Design review of the part shown in the three views and the two pictorial views. Dimensions are in mm from the part's minimum x, y and z. A direction names the side the tool comes from. Round coordinates to 2 decimals unless told otherwise and drop trailing zeros. Loops run counter-clockwise (first coordinate to the right, second up) from the corner with the lowest first, then second, coordinate; pieces in that order, holes last. Notation, with made-up numbers: M 41.5,72 L 61.5,72 A37 cw 61.5,109 Z; hole C -39,70.5 d8. An arc over 180 degrees is marked long. One line per question, with ' | ' between items.
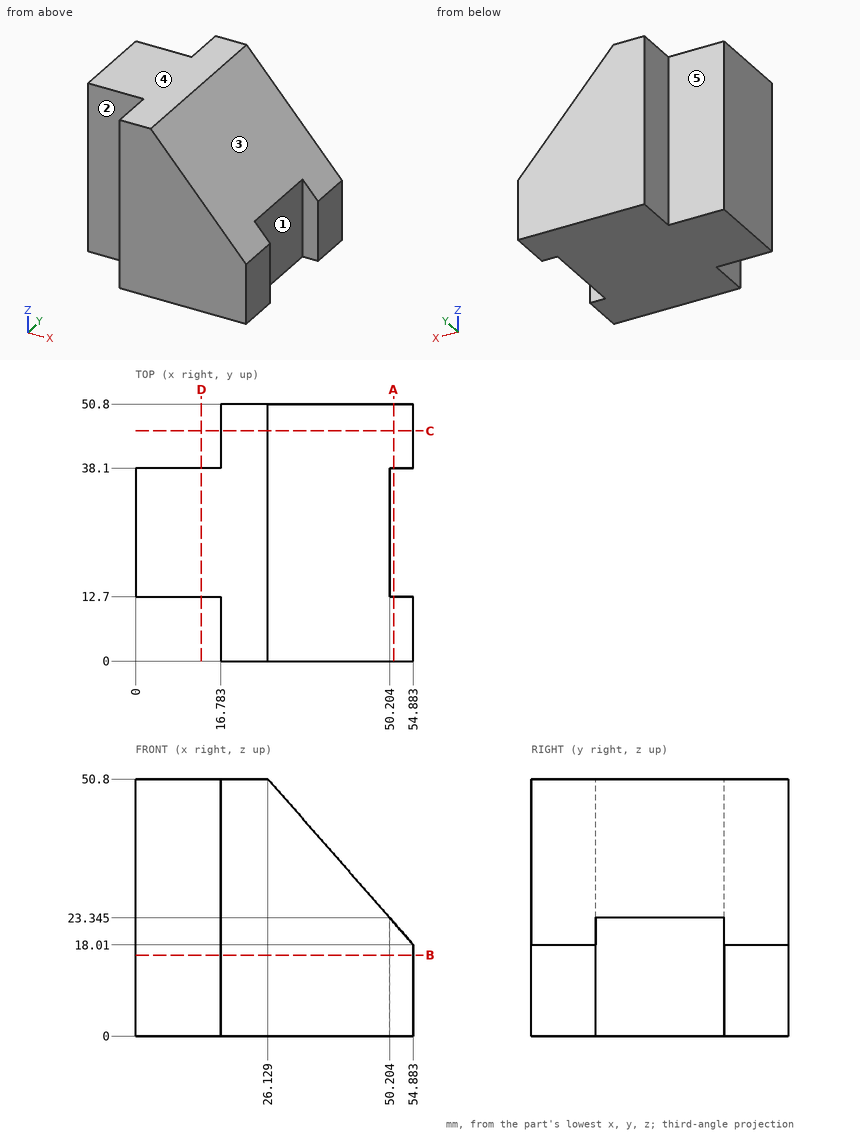
1) Add section C-C on y = 45.5. State the section outline as (x, z) points.
Output values:
outline: M 16.78,0 L 54.88,0 L 54.88,18.01 L 26.13,50.8 L 16.78,50.8 Z
2) Add section B-B on z = 16. State the section outline as (x, y) points, then the cut area to 3 significant figures.
Output values:
outline: M 0,12.7 L 16.78,12.7 L 16.78,0 L 54.88,0 L 54.88,12.7 L 50.2,12.7 L 50.2,38.1 L 54.88,38.1 L 54.88,50.8 L 16.78,50.8 L 16.78,38.1 L 0,38.1 Z | area: 2,240 mm²
3) Machinability: for the marked faces 4 and 5, which of the approach directions +Z, -Z, +X, -X, +Y, -Y give a long, thin tool a straight path to every point of the face, cutting with its end or side? Answer none if there is none.
Output values:
face 4: +Z, +X, -X, +Y, -Y | face 5: +Z, -Z, -X, +Y
4) Add section D-D on x = 13. State the section outline as (y, z) points, then the cut area to 3 significant figures.
Output values:
outline: M 12.7,0 L 38.1,0 L 38.1,50.8 L 12.7,50.8 Z | area: 1,290 mm²
5) Add section A-A on x = 51. State the section outline as (y, z) points, then the cut area to 3 significant figures.
Output values:
outline: M 0,0 L 12.7,0 L 12.7,22.44 L 0,22.44 Z; M 38.1,0 L 50.8,0 L 50.8,22.44 L 38.1,22.44 Z | area: 570 mm²
6) Insertion check: P1, Ø18.5, axis at y = 26, z = 15.5, coming from the +X side; P2, Ø10, axis at x = 9.5, z = 34.5, coming from the -Y side; P3, Ø1, axis at x = 42.5, y = 39.5, coming from the +Z side. Each pin has a flat end and moves straight along its axis. Give the tip position at first contact, or say it passes through.
Output values:
P1: stops at x = 50.2 | P2: stops at y = 12.7 | P3: stops at z = 32.7
7) For line 1 (X direction, y = 40.5, z = 12); line 2 (Y direction, x = 7, z = 6); line 3 (X direction, y = 16.5, z = 14.5), list the stretches that pass through material, from the lowest coordinate up.
Output values:
line 1: x = 16.78 to 54.88 | line 2: y = 12.7 to 38.1 | line 3: x = 0 to 50.2
8) Mouldability with a two-part tool opening along Y and no side actions: class the marked faces 1, 2 and 3 as +Y half, -Y half, draft (parallel to the pull), parting line (faces both ways), or undercut.
Output values:
face 1: undercut | face 2: -Y half | face 3: draft
